Work out the finished part from the listing and answer in its coordinate system (mm). Round coordinates to 2 decimals unless told otherwise and drop trailing zeros. Write each loop counter-clockwise with the first axis right and the second up, starting at its lowest first coordinate (ties: lowest second). Pieces come first, ordered by that corner, then holes. Notation, with made-up numbers: M 42.25,-25.75 L 88.25,-25.75 A26 ccw 88.25,-5.75 Z; hole C 21.5,-20.5 d1. An arc over 180 degrees is marked long. Answer in a Markdown table with one row per item.
```python
from build123d import *

# Parameters (mm, degrees)
SKETCH_1_W          = 41
SKETCH_1_H          = 60
EXTRUDE_1_DEPTH     = 3
SKETCH_2_R          = 1.75
CUT_EXTRUDE_1_DEPTH = 3
FILLET_1_R          = 2
CHAMFER_2_SIZE      = 1
CHAMFER_1_SIZE      = 2
CHAMFER_3_SIZE      = 0.5


with BuildPart() as part:
    # Эскиз1 → Бобышка-Вытянуть1 (new body)
    with BuildSketch(Plane(origin=(0, 0, 0), x_dir=(1, 0, 0), z_dir=(0, 1, 0))):
        Rectangle(SKETCH_1_W, SKETCH_1_H)
    extrude(amount=EXTRUDE_1_DEPTH)

    # Эскиз2 → Вырез-Вытянуть1 (cut)
    with BuildSketch(Plane(origin=(0, 3, 0), x_dir=(1, 0, 0), z_dir=(0, 1, 0))):
        with Locations(Location((16, 18, 0), (0, 0, 270))):
            Circle(SKETCH_2_R)
        with Locations(Location((16, -18, 0), (0, 0, 90))):
            Circle(SKETCH_2_R)
        with Locations(Location((-16, -18, 0), (0, 0, 270))):
            Circle(SKETCH_2_R)
        with Locations(Location((-16, 18, 0), (0, 0, 90))):
            Circle(SKETCH_2_R)
    extrude(amount=-CUT_EXTRUDE_1_DEPTH, mode=Mode.SUBTRACT)

    # Скругление1
    fillet_1_edges = [part.edges().sort_by_distance(p)[0] for p in [
        (20.5, 1.5, 30),
        (-20.5, 1.5, 30),
        (-20.5, 1.5, -30),
        (20.5, 1.5, -30),
    ]]
    fillet(fillet_1_edges, radius=FILLET_1_R)

    # Фаска2
    chamfer_2_edges = [part.edges().sort_by_distance(p)[0] for p in [
        (0, 3, -30),
        (20.5, 3, 0),
        (-20.5, 3, 0),
        (0, 3, 30),
        (19.914213562, 3, 29.414213562),
        (-19.914213562, 3, 29.414213562),
        (-19.914213562, 3, -29.414213562),
        (19.914213562, 3, -29.414213562),
    ]]
    chamfer(chamfer_2_edges, length=CHAMFER_2_SIZE)

    # Фаска1
    # the kernel refuses this chamfer: 2 mm, written as the material it takes off along each edge
    with BuildSketch(Plane(origin=(-16, 3, -18), x_dir=(0, 0, -1), z_dir=(1, 0, 0))) as chamfer_1_piece_1:
        Polygon((1.75 + CHAMFER_1_SIZE, 0), (1.75, -CHAMFER_1_SIZE), (1.75, 0), align=None)
    revolve(axis=Axis((-16, 3, -18), (0, 1, 0)), mode=Mode.SUBTRACT)
    with BuildSketch(Plane(origin=(-16, 3, 18), x_dir=(0, 0, 1), z_dir=(-1, 0, 0))) as chamfer_1_piece_2:
        Polygon((1.75 + CHAMFER_1_SIZE, 0), (1.75, -CHAMFER_1_SIZE), (1.75, 0), align=None)
    revolve(axis=Axis((-16, 3, 18), (0, 1, 0)), mode=Mode.SUBTRACT)
    with BuildSketch(Plane(origin=(16, 3, 18), x_dir=(0, 0, -1), z_dir=(1, 0, 0))) as chamfer_1_piece_3:
        Polygon((1.75 + CHAMFER_1_SIZE, 0), (1.75, -CHAMFER_1_SIZE), (1.75, 0), align=None)
    revolve(axis=Axis((16, 3, 18), (0, 1, 0)), mode=Mode.SUBTRACT)
    with BuildSketch(Plane(origin=(16, 3, -18), x_dir=(0, 0, 1), z_dir=(-1, 0, 0))) as chamfer_1_piece_4:
        Polygon((1.75 + CHAMFER_1_SIZE, 0), (1.75, -CHAMFER_1_SIZE), (1.75, 0), align=None)
    revolve(axis=Axis((16, 3, -18), (0, 1, 0)), mode=Mode.SUBTRACT)

    # Фаска3
    chamfer_3_edges = [part.edges().sort_by_distance(p)[0] for p in [
        (-16, 0, -16.25),
        (-16, 0, 16.25),
        (16, 0, 19.75),
        (16, 0, -19.75),
        (0, 0, -30),
        (20.5, 0, 0),
        (0, 0, 30),
        (-20.5, 0, 0),
        (19.914213562, 0, 29.414213562),
        (-19.914213562, 0, 29.414213562),
        (-19.914213562, 0, -29.414213562),
        (19.914213562, 0, -29.414213562),
    ]]
    chamfer(chamfer_3_edges, length=CHAMFER_3_SIZE)


solid = part.part
```
1. The part is cut by section B-B (z = -18). Determine the outline of the cut face in (x, y) (3 decimals), plus the area to 3 significant figures.
Calculated:
| item | result |
|---|---|
| outline | M -20.5,0.5 L -20,0 L -18.25,0 L -17.75,0.5 L -17.75,1 L -19.625,2.875 L -20.5,2 Z; M -14.25,0.5 L -13.75,0 L 13.75,0 L 14.25,0.5 L 14.25,1 L 12.25,3 L -12.25,3 L -14.25,1 Z; M 17.75,0.5 L 18.25,0 L 20,0 L 20.5,0.5 L 20.5,2 L 19.625,2.875 L 17.75,1 Z |
| area | 92.3 mm² |
2. The part is cut by section A-A (x = -16). Determine the outline of the cut face in (y, z), plus the area to 3 significant figures.
Calculated:
| item | result |
|---|---|
| outline | M 0,-29.5 L 0.5,-30 L 2,-30 L 3,-29 L 3,-21.75 L 1,-19.75 L 0.5,-19.75 L 0,-20.25 Z; M 0,-15.75 L 0.5,-16.25 L 1,-16.25 L 3,-14.25 L 3,14.25 L 1,16.25 L 0.5,16.25 L 0,15.75 Z; M 0,20.25 L 0.5,19.75 L 1,19.75 L 3,21.75 L 3,29 L 2,30 L 0.5,30 L 0,29.5 Z |
| area | 149 mm² |
3. Determine the mould class of faces 1 (the cylindrical face through (-17.735, 0.753, -17.772)), 2 (the flat face through (0, 0, 0)), 3 (the cylindrical face through (17.735, 0.753, -18.228)), 4 (the conical face through (-19.48, 2.6, 29)) for opening direction X: released by +X, released by -X, zero draft, split by the parting line, or undercut.
Calculated:
| item | result |
|---|---|
| face 1 | undercut |
| face 2 | zero draft |
| face 3 | undercut |
| face 4 | released by -X |
4. Given pin 1 (4 mm diameter, centred on x = 16, z = 18, fed in from +Y); pin 2 (5.5 mm diameter, centred on x = -16, z = -18, fed in from +Y), each flat-ended and moving along its own axis, determine where each tip first touches the part or whether it passes through.
Calculated:
| item | result |
|---|---|
| pin 1 | stops at y = 1.25 |
| pin 2 | stops at y = 2 |
5. The part is cut by section C-C (x = 17). Count the separate pieces of the cut face and the enclosed holes in it, plus the area to 3 significant figures.
Calculated:
| item | result |
|---|---|
| separate pieces | 3 |
| enclosed holes | 0 |
| area | 152 mm² |
6. Consider line 1 along X through (y, z) = (0.8, 18); line 2 along X through (y, z) = (0.75, -19.5); line 3 along Z through (x, y) = (15, 1.85). Determine where each line is inside the solid, lowest interval first. Write a range as from..to.
Calculated:
| item | result |
|---|---|
| line 1 | x = -20.5..-17.75, -14.25..14.25, 17.75..20.5 |
| line 2 | x = -20.5..-16.9, -15.1..15.1, 16.9..20.5 |
| line 3 | z = -30..-20.4, -15.6..15.6, 20.4..30 |
